Autodesk Inventor part; units mm, degrees
ref_plane "Work Plane1" through (0, 0, 40) normal (0, 0, 1) x (1, 0, 0)
ref_plane "YZ Plane" through (0, 0, 0) normal (1, 0, 0) x (0, 1, 0)
ref_plane "XZ Plane" through (0, 0, 0) normal (0, 1, 0) x (-1, 0, 0)
sketch "Sketch1" plane through (0, 0, 0) normal (0, 0, 1) x (1, 0, 0)
  circle A0 centre (0, 0) radius 500
  dimension "d0" = 1000
extrude "Extrusion1" add sketch "Sketch1" along normal blind 40
ref_plane "Work Plane1" through (0, 0, 40) normal (0, 0, 1) x (1, 0, 0)
sketch "Sketch2" plane through (0, 0, 40) normal (0, 0, 1) x (1, 0, 0)
  circle A0 centre (0, 400) radius 40
  circle A1 centre (400, 0) radius 40
  circle A2 centre (0, -400) radius 40
  circle A3 centre (-400, 0) radius 40
  point P0 (0, 0)
  dimension "d4" = 80
  dimension "d5" = 80
  dimension "d6" = 80
  dimension "d7" = 80
  dimension "d8" = 400
  dimension "d9" = 400
  dimension "d10" = 400
  dimension "d11" = 400
extrude "Extrusion2" add sketch "Sketch2" along normal blind 800
properties part number "Maitri_table"
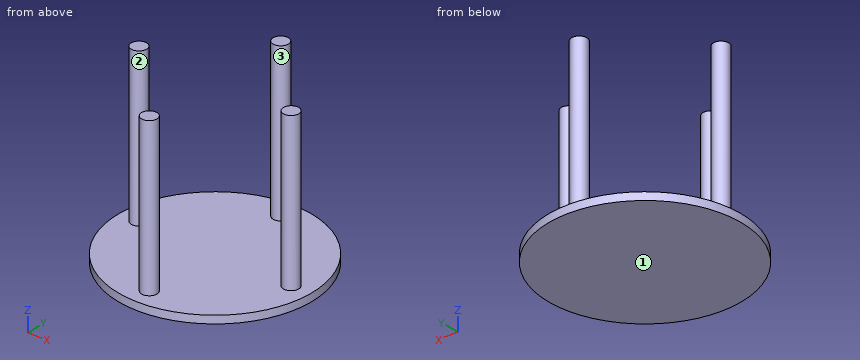
The listing builds one solid part. Answer for the finished solid, in the listing's coordinates (mm). Face numbers are marked on the shaded views. Round coordinates to 2 decimals unless told otherwise and drop trailing zeros. Write each loop counter-clockwise with the first axis right and the second up, starting at its lowest first coordinate (ties: lowest second). Pieces come first, ordered by that corner, then holes. Notation, with made-up numbers: (86.25, 88.5) -> (140.25, 88.5) arc R22 cw to (140.25, 110.5) -> close; hole circle Ø2 at (16.25, -14.5). An arc over 180 degrees is marked (long way). Answer as a JSON object with one key per item and string values. Group by question number.
Q1. Section C-C (z = 214.5) is taken. Write down the section's boundary in (x, y).
Q2. Determine the mould class of the marked faces 1, 2 and 3 for opening direction Y: pulls with the +Y half, pulls with the -Y half, needs draft (parallel to the pull), parting line crosses it, or undercut.
Q3. Section A-A (x = 0) is taken. Write down the section's boundary in (y, z), plus the area to 3 significant figures.
Q4. Straight lines are drawn through the part: line 1 along Z through (x, y) = (398, -277); line 2 along Y through (x, z) = (-1.5, 749); line 3 along Y through (x, z) = (-436.5, 601). For each, find the intervals that lie inside material, in ascending order.
Q5. Section D-D (x = 411) is taken. Write down the section's boundary in (y, z), plus the area to 3 significant figures.
Q6. Each of these flat-tipped pins is pushed along its axis until it touches: pin 1 Ø10 at (y, z) = (-20, 154.5) entering from +X; pin 2 Ø12 at (x, z) = (352.5, 584.5) entering from -Y. Where does it stop, or does it pass through?
Q7. Section B-B (y = 400) is taken. Write down the section's boundary in (x, z).
Check values:
{
 "1": {"outline": "circle Ø80 at (-400, 0); circle Ø80 at (0, -400); circle Ø80 at (0, 400); circle Ø80 at (400, 0)"},
 "2": {"face 1": "needs draft", "face 2": "parting line crosses it", "face 3": "undercut"},
 "3": {"outline": "(-500, 0) -> (500, 0) -> (500, 40) -> (440, 40) -> (440, 840) -> (360, 840) -> (360, 40) -> (-360, 40) -> (-360, 840) -> (-440, 840) -> (-440, 40) -> (-500, 40) -> close", "area": "168,000 mm^2"},
 "4": {"line 1": "0 to 40", "line 2": "-439.97 to -360.03, 360.03 to 439.97", "line 3": "-16.36 to 16.36"},
 "5": {"outline": "(-284.74, 0) -> (284.74, 0) -> (284.74, 40) -> (38.46, 40) -> (38.46, 840) -> (-38.46, 840) -> (-38.46, 40) -> (-284.74, 40) -> close", "area": "84,300 mm^2"},
 "6": {"pin 1": "x = 437.08", "pin 2": "through"},
 "7": {"outline": "(-300, 0) -> (300, 0) -> (300, 40) -> (40, 40) -> (40, 840) -> (-40, 840) -> (-40, 40) -> (-300, 40) -> close"}
}
